Autodesk Inventor part; units mm, degrees
ref_plane "YZ Plane" through (0, 0, 0) normal (1, 0, 0) x (0, 1, 0)
ref_plane "XZ Plane" through (0, 0, 0) normal (0, 1, 0) x (-1, 0, 0)
ref_plane "XY Plane" through (0, 0, 0) normal (0, 0, 1) x (1, 0, 0)
sketch "Sketch1" plane through (0, 0, 0) normal (0, 1, 0) x (-1, 0, 0)
  line L0 (-12.7, -12.7) -> (10.45, -12.7)
  line L1 (12.7, -10.45) -> (12.7, 12.7)
  line L2 (12.7, 12.7) -> (-12.7, 12.7)
  line L3 (-12.7, 12.7) -> (-12.7, -12.7)
  line L4 (-12.7, -12.7) -> (12.7, 12.7) construction
  line L5 (12.7, -12.7) -> (-12.7, 12.7) construction
  line L6 (17.473, -17.473) -> (23.3066, -23.3066)
  arc A0 (14.291, -17.473) -> (17.473, -14.291) centre (15.882, -15.882) ccw
  line L7 (14.291, -11.109) -> (17.473, -14.291)
  line L8 (11.109, -14.291) -> (14.291, -17.473)
  line L9 (12.7, -10.45) -> (12.7, -12.7)
  line L10 (12.7, -12.7) -> (10.45, -12.7)
  arc A1 (14.291, -11.109) -> (12.7, -10.45) centre (12.7, -12.7) ccw
  arc A2 (10.45, -12.7) -> (11.109, -14.291) centre (12.7, -12.7) ccw
  point P0 (0, 0)
  point P1 (15.882, -15.882)
  dimension "d0" = 25.4
extrude "Extrusion1" add sketch "Sketch1" along normal blind 45 contours L10 L9 A1 L7 A0 L8 A2
sketch "Sketch2" plane through (0, 45, 0) normal (0, 1, 0) x (1, 0, 0)
  arc A0 (-14.291, 11.109) -> (-12.7, 10.45) centre (-12.7, 12.7) ccw
  line L0 (-12.7, 10.45) -> (-12.7, 12.7)
  line L1 (-12.7, 12.7) -> (-10.45, 12.7)
  arc A1 (-10.45, 12.7) -> (-11.109, 14.291) centre (-12.7, 12.7) ccw
  line L2 (-11.109, 14.291) -> (-14.291, 17.473)
  arc A2 (-14.291, 17.473) -> (-17.473, 14.291) centre (-15.882, 15.882) ccw
  line L3 (-17.473, 14.291) -> (-14.291, 11.109)
  line L4 (-17.473, 17.473) -> (-15.882, 19.064)
  arc A3 (-14.291, 17.473) -> (-17.473, 14.291) centre (-15.882, 15.882) ccw
  line L5 (-15.882, 19.064) -> (-19.064, 15.882)
  line L6 (-19.064, 15.882) -> (-14.291, 11.109)
  line L7 (-14.291, 11.109) -> (-11.109, 14.291)
  line L8 (-11.109, 14.291) -> (-15.882, 19.064)
  line L9 (-19.064, 15.882) -> (-26.135, 22.953)
  line L10 (-15.882, 19.064) -> (-22.953, 26.135)
  line L11 (-22.953, 26.135) -> (-26.135, 22.953)
  point P0 (0, 0)
  dimension "d10" = 10
extrude "Extrusion2" add sketch "Sketch2" against normal blind 9 contours L3 A2 L2 L7 | L6 L5 A2 | L4 L8 A2 | L5 L9 L11 L10 L4
sketch "Sketch3" plane through (-22.953, 36, -26.135) normal (-0.7071, 0, -0.7071) x (-0.7071, 0, 0.7071)
  line L0 (0, 0) -> (4.5, 0)
  line L1 (4.5, 9) -> (4.5, 0)
  line L2 (4.5, -36) -> (4.5, 9)
  line L3 (0, 9) -> (4.5, 9)
  line L4 (4.25, 2.2514) -> (4.75, 2.2514)
  line L5 (4.75, 2.2514) -> (4.75, 6.7486)
  line L6 (4.75, 6.7486) -> (4.25, 6.7486)
  line L7 (4.25, 6.7486) -> (4.25, 2.2514)
  line L8 (4.25, 2.2514) -> (4.75, 6.7486) construction
  line L9 (4.75, 2.2514) -> (4.25, 6.7486) construction
  line L10 (-0.25, 2) -> (0.25, 2)
  line L11 (0.25, 2) -> (0.25, 7)
  line L12 (0.25, 7) -> (-0.25, 7)
  line L13 (-0.25, 7) -> (-0.25, 2)
  line L14 (0, -36) -> (0, 9)
  line L15 (-0.25, 2) -> (0.25, 7) construction
  line L16 (0.25, 2) -> (-0.25, 7) construction
  line L17 (4.5, 6.7486) -> (4.5, 2.2514)
  line L18 (0, 2) -> (0, 7)
  point P0 (2.25, -36)
  point P1 (4.5, 4.5)
  point P2 (0, 4.5)
  dimension "d13" = 9
  dimension "d14" = 4.5
  dimension "d15" = 4.5
  dimension "d16" = 0.5
  dimension "d17" = 0.5
  dimension "d18" = 5
extrude "Extrusion3" cut sketch "Sketch3" against normal blind 21.7 contours L14 L12 L11 L10 | L10 L13 L12 L14 | L4 L7 L6 L1 | L1 L6 L5 L4
properties part number "Gripper_Gen3_FingerRail"
For this review, take the finished solid that the model builds, in its own axes (mm). A direction names the side the tool comes from. Give positions to 0.01 mm unless a question says otherwise; leave off trailing zeros. Loops run counter-clockwise (first coordinate to the right, second up) from the corner with the lowest first, then second, coordinate; pieces in that order, holes last. Notation, with made-up numbers: M -10.5,-0.75 L 11.5,-0.75 A29 ccw 11.5,26.25 Z; hole C 22.25,-22.75 d1. An arc over 180 degrees is marked long. One line per item, written item: value. Start each with the question number.
Q1. For L1, parallel to Y at x = -21.25, z = -18.25; L2, parallel to Y at x = -17.5, z = -19.75; L3, parallel to X at y = 17, z = -15, list the stretches that pass through material, from the lowest coordinate up.
Q2. Add section A-A (y = 41). Give the boundary of the cut face in (x, z), and give its area (3 significant figures).
Q3. Machinability: for faces 1 (the face through (-17.508, 17.748, -17.438)), 2 (the face through (-12.7, 22, -12)), 3 (the face through (-16.93, 40.47, -19.76)), 4 (the face through (-10.626, 22.185, -13.572)), which of the approach directions +Z, -Z, +X, -X, +Y, -Y give a long, thin tool a straight path to every point of the face, cutting with its end or side? Answer none if there is none.
Q4. Add section C-C (z = -12). Give the boundary of the cut face in (x, y), and give its area (3 significant figures).
Q5. Add section B-B (x = -16). Give the boundary of the cut face in (y, z).
Q6. Clearance check with flat-ended pins moving along their axes: pin 1 Ø2 at (x, y) = (-14, 15) entering from -Z; pin 2 Ø1.8 at (x, y) = (-12, 30.5) entering from +Z; pin 3 Ø4 at (x, y) = (-14, 32) entering from -Z; pin 4 Ø4 at (x, z) = (-17.5, -20) entering from -Y. State where each tip first meets the part, or that it passes through.
Q7. Draft analysis for pull direction Y (two halves, no side actions). For faces 5 (the face through (-19.76, 40.53, -16.93)), 6 (the face through (-15, 0, -15)), 7 (the face through (-13.494, 20.319, -16.676)), state which applies: released by +Y, released by -Y, zero draft, split by the parting line, or undercut.
Reply:
1. L1: 36 to 38.25, 42.75 to 45
1. L2: 36 to 45
1. L3: -17.95 to -11.82
2. outline: M -25.96,-23.13 L -23.13,-25.96 L -10.56,-13.39 A2.25 ccw -10.45,-12.7 L -12.7,-12.7 L -12.7,-10.45 A2.25 ccw -13.39,-10.56 Z
2. area: 70.6 mm²
3. face 1: -Y
3. face 2: +Z, +X, +Y, -Y
3. face 3: -Z, +X
3. face 4: -Z, +X, +Y, -Y
4. outline: M -15.18,0 L -12.7,0 L -12.7,45 L -15.18,45 L -15.18,42.75 L -14.83,42.75 L -14.83,38.25 L -15.18,38.25 Z
4. area: 110 mm²
5. outline: M 0,-18.13 L 36,-18.13 L 36,-19.18 L 38,-19.18 L 38,-18.83 L 43,-18.83 L 43,-19.18 L 45,-19.18 L 45,-12.82 L 42.75,-12.82 L 42.75,-13.17 L 38.25,-13.17 L 38.25,-12.82 L 0,-12.82 Z
6. pin 1: z = -17.95
6. pin 2: z = -10.45
6. pin 3: z = -18.13
6. pin 4: y = 36
7. face 5: undercut
7. face 6: released by -Y
7. face 7: zero draft
